Could you check a few things on this model? Use its own coordinates, in mm. A direction names the side the tool comes from. Give positions to 0.01 mm unless a question says otherwise; leave off trailing zeros. Loops run counter-clockwise (first coordinate to the right, second up) from the corner with the lowest first, then second, coordinate; pieces in that order, holes last.
1. Imagine slicing it at B-B (y = 15). List the corners of the cut face in (x, z) for me.
2. For P1, Ø1.8, axis at x = -55, y = 15, coming from the +Z side; P2, Ø4, axis at x = -55, y = -20, coming from the -Z side, each with a flat end and sliding along its axis, tell me the tip position at first contact or that it passes through.
3. Imagine slicing it at A-A (x = -55). List the corners of the cut face in (y, z) for me, plus the area to 3 significant figures.
4. Imagine slicing it at D-D (z = 2.45). List the corners of the cut face in (x, y) for me, plus the area to 3 significant figures.
5. For faces 1 (the flat face through (0, -20, 1)), 2 (the flat face through (-1, -25, 1)), which set-ups out of +Z, -Z, +X, -X, +Y, -Y let a thin tool reach every point of the face, with its end or its side?
6. Thinking about a two-plate mould opening in X: for faces 3 (the flat face through (-20, -5, 1)), 4 (the flat face through (-1, 11, 0)), 5 (the flat face through (-60, 0, 1)), 6 (the cylindrical face through (53.57, -20.45, 1.48)), which applies, +X half, -X half, draft (parallel to the pull), parting line (faces both ways), or undercut?
7. Imagine slicing it at C-C (y = -13). List the corners of the cut face in (x, z) for me.
8. I need wall thicknesses on line 1 along X through (y, z) = (-14, 0.5); line 2 along Y through (x, z) = (55, 1.1); line 3 along Y through (x, z) = (17, 1.15). Which ranges of each line are inside material? Lowest first, please.
```python
from build123d import *

# Parameters (mm, degrees)
ESQUISSE1_W        = 120
ESQUISSE1_H        = 50
ESQUISSE1_R        = 1.5
ESQUISSE1_W_2      = 40
ESQUISSE1_H_2      = 30
BOSS_EXTRU_1_DEPTH = 3


with BuildPart() as part:
    # Esquisse1 → Boss.-Extru.1 (new body)
    with BuildSketch(Plane.XY):
        Rectangle(ESQUISSE1_W, ESQUISSE1_H)
        with Locations((-55, 15)):
            Circle(ESQUISSE1_R, mode=Mode.SUBTRACT)
        with Locations((-55, -20)):
            Circle(ESQUISSE1_R, mode=Mode.SUBTRACT)
        with Locations(Location((55, -20, 0), (0, 0, 180))):
            Circle(ESQUISSE1_R, mode=Mode.SUBTRACT)
        with Locations(Location((55, 15, 0), (0, 0, 180))):
            Circle(ESQUISSE1_R, mode=Mode.SUBTRACT)
        with Locations((0, -5)):
            Rectangle(ESQUISSE1_W_2, ESQUISSE1_H_2, mode=Mode.SUBTRACT)
    extrude(amount=BOSS_EXTRU_1_DEPTH)


solid = part.part
```
Derived:
1. outline: (-60, 0) - (-56.5, 0) - (-56.5, 3) - (-60, 3) - close; (-53.5, 0) - (53.5, 0) - (53.5, 3) - (-53.5, 3) - close; (56.5, 0) - (60, 0) - (60, 3) - (56.5, 3) - close
2. P1: passes through
2. P2: stops at z = 0
3. outline: (-25, 0) - (-21.5, 0) - (-21.5, 3) - (-25, 3) - close; (-18.5, 0) - (13.5, 0) - (13.5, 3) - (-18.5, 3) - close; (16.5, 0) - (25, 0) - (25, 3) - (16.5, 3) - close
3. area: 132 mm2
4. outline: (-60, -25) - (60, -25) - (60, 25) - (-60, 25) - close; hole circle Ø3 at (-55, -20); hole circle Ø3 at (-55, 15); hole (-20, -20) - (20, -20) - (20, 10) - (-20, 10) - close; hole circle Ø3 at (55, -20); hole circle Ø3 at (55, 15)
4. area: 4,770 mm2
5. face 1: +Z, -Z
5. face 2: +Z, -Z, +X, -X, -Y
6. face 3: undercut
6. face 4: draft
6. face 5: -X half
6. face 6: undercut
7. outline: (-60, 0) - (-20, 0) - (-20, 3) - (-60, 3) - close; (20, 0) - (60, 0) - (60, 3) - (20, 3) - close
8. line 1: x = -60 to -20, 20 to 60
8. line 2: y = -25 to -21.5, -18.5 to 13.5, 16.5 to 25
8. line 3: y = -25 to -20, 10 to 25
